Can you work these out from the model? Positions are in its coordinate system, mm. A direction names the side the tool comes from. Round coordinates to 2 decimals unless told otherwise and drop trailing zeros. Write each loop counter-clockwise with the first axis right and the second up, starting at its lowest first coordinate (ties: lowest second). Pieces come first, ordered by that corner, then holes.
Q1. If we section it at B-B (x = 114): Please give me the cut outline in (y, z), plus the area to 3 significant figures.
Q2. We'd pull the mould along X, two halves only. Please class faces 4 (the flat face through (-0.838, -174, 3)), 5 (the cylindrical face through (129.027, -479.204, 11.201)), 6 (the conical face through (123.55, -417.47, -147.82)): +X half, -X half, draft (parallel to the pull), parting line (faces both ways), or undercut.
Q3. For faces 1 (the cylindrical face through (63.72, -466.517, 10.643)), 2 (the cylindrical face through (66.1, -237.377, 0.558)), 3 (the cylindrical face through (-2.598, -469.622, 10.78)), which set-ups out of +Z, -Z, +X, -X, +Y, -Y let a thin tool reach every point of the face, with its end or its side?
Q4. I'm going to push flat-ended pins straight in: pin 1 Ø4 at (x, y) = (74.5, -352.5) entering from -Z; pin 2 Ø20.5 at (y, z) = (-224.69, 0) entering from +X; pin 3 Ø6 at (x, y) = (52.5, -83.5) entering from -Z; pin 4 Ø2 at (x, z) = (80.5, 149) entering from +Y. Where does each tip first touch, or does it pass through?
Q5. Please list where these lines run through material, in increasing order: line 1 along X through (y, z) = (-353, -107.5); line 2 along Z through (x, y) = (6.5, -227); line 3 along Z through (x, y) = (28.5, -50).
from build123d import *

# Parameters (mm, degrees)
F2_R     = 12.7
F3_DEPTH = 134.8161187441


# Not quite as in the source:
# - a feature names something its author has since deleted; it is built from what else it names


with BuildPart() as f1:
    # F0 (on Top) → F1 (revolve)
    with BuildSketch(Plane.XY):
        with BuildLine():
            Line((-3.6245174784, 29.0860664694), (-3.6245174784, 20.4818164694))
            Line((-3.6245174784, 20.4818164694), (-1.6004623353, 20.4818164694))
            ThreePointArc((-1.6004623353, 20.4818164694), (-1.0616469681, 20.2586318366), (-0.8384623353, 19.7198164694))
            Line((-0.8384623353, 19.7198164694), (-0.8384623353, -224.6888160382))
            Line((-0.8384623353, -224.6888160382), (131.1906012657, -224.6888160382))
            Line((131.1906012657, -224.6888160382), (131.1906012657, 29.3111839618))
            ThreePointArc((131.1906012657, 29.3111839618), (130.967416633, 29.8499993291), (130.4286012657, 30.0731839618))
            Line((130.4286012657, 30.0731839618), (127.6640418936, 30.0731839618))
            Line((127.6640418936, 30.0731839618), (123.3422697523, 17.6397553064))
            ThreePointArc((123.3422697523, 17.6397553064), (123.1973905872, 17.4466211557), (122.967395476, 17.3731839618))
            Line((122.967395476, 17.3731839618), (6.1083994667, 17.3731839618))
            ThreePointArc((6.1083994667, 17.3731839618), (5.8880446333, 17.4399778914), (5.7418610892, 17.6178768884))
            Line((5.7418610892, 17.6178768884), (0.6640418936, 29.8480664694))
            Line((0.6640418936, 29.8480664694), (-2.8625174784, 29.8480664694))
            ThreePointArc((-2.8625174784, 29.8480664694), (-3.4013328457, 29.6248818366), (-3.6245174784, 29.0860664694))
        make_face()
    revolve(axis=Axis((65.1760694652, -224.6888160382, 0), (1, 0, 0)))

    # F2 (on face) → F3 (cut, through all)
    with BuildSketch(Plane.YZ.offset(131.1906012657)):
        with Locations((-224.6888160382, 0)):
            Circle(F2_R)
    extrude(amount=-F3_DEPTH, mode=Mode.SUBTRACT)


solid = f1.part
A:
1. outline: circle Ø484.12 at (-224.69, 0); hole circle Ø25.4 at (-224.69, 0)
1. area: 184,000 mm2
2. face 4: -X half
2. face 5: draft
2. face 6: undercut
3. face 1: none
3. face 2: +X, -X
3. face 3: -X
4. pin 1: stops at z = -206.8
4. pin 2: passes through
4. pin 3: stops at z = -198.74
4. pin 4: stops at y = -33.14
5. line 1: x = -0.84 to 131.19
5. line 2: z = -242.05 to -12.49, 12.49 to 242.05
5. line 3: z = -167.56 to 167.56
